from build123d import *

# Parameters (mm, degrees)
BOSS_EXTRUDE1_DEPTH      = 3
SKETCH2_W                = 3
SKETCH2_H                = 34
BOSS_EXTRUDE2_DEPTH      = 17
BOSS_EXTRUDE2_DEPTH_BACK = 3
SKETCH3_W                = 22.5
SKETCH3_H                = 29.060921084
CUT_EXTRUDE1_DEPTH       = 18
CUT_EXTRUDE2_DEPTH       = 1.5
CHAMFER1_SIZE            = 10
CHAMFER2_SIZE            = 1.5
CHAMFER2_SIZE2           = 2.223841453
SKETCH7_W                = 31
SKETCH7_H                = 2
BOSS_EXTRUDE3_DEPTH      = 2
BOSS_EXTRUDE3_DEPTH_BACK = 3
SKETCH9_W                = 0.5
SKETCH9_H                = 11.560921084
CUT_EXTRUDE4_DEPTH       = 10
CHAMFER3_SIZE            = 1.5
CUT_EXTRUDE6_START       = -16.5
SKETCH11_W               = 3
SKETCH11_H               = 5
CUT_EXTRUDE6_DEPTH       = 16.5
CHAMFER9_SIZE            = 2
CHAMFER10_SIZE           = 3.5
FILLET2_R                = 2


with BuildPart() as part:
    # Sketch1 → Boss-Extrude1 (new body)
    with BuildSketch(Plane.XY):
        with BuildLine():
            Line((38, 38.915798387), (-38, 38.915798387))
            Line((-38, 38.915798387), (-38, 9.854877303))
            Line((-38, 9.854877303), (-34.5, 9.854877303))
            Line((-34.5, 9.854877303), (-34.5, 15.915798387))
            Line((-34.5, 15.915798387), (-34.5, 21.415798387))
            Line((-34.5, 21.415798387), (-29, 21.415798387))
            Line((-29, 21.415798387), (-21, 21.415798387))
            ThreePointArc((-21, 21.415798387), (-17.110912703, 19.804885683), (-15.5, 15.915798387))
            Line((-15.5, 15.915798387), (-15.5, 9.854877303))
            Line((-15.5, 9.854877303), (15.5, 9.854877303))
            Line((15.5, 9.854877303), (15.5, 15.915798387))
            ThreePointArc((15.5, 15.915798387), (17.110912703, 19.804885683), (21, 21.415798387))
            Line((21, 21.415798387), (29, 21.415798387))
            ThreePointArc((29, 21.415798387), (32.889087297, 19.804885683), (34.5, 15.915798387))
            Line((34.5, 15.915798387), (34.5, 9.854877303))
            Line((34.5, 9.854877303), (38, 9.854877303))
            Line((38, 9.854877303), (38, 38.915798387))
        make_face()
        with BuildLine():
            Line((-10.5, 33.665798387), (-5.5, 33.665798387))
            ThreePointArc((-5.5, 33.665798387), (-3.75, 31.915798387), (-5.5, 30.165798387))
            Line((-5.5, 30.165798387), (-10.5, 30.165798387))
            ThreePointArc((-10.5, 30.165798387), (-12.25, 31.915798387), (-10.5, 33.665798387))
        make_face(mode=Mode.SUBTRACT)
        with BuildLine():
            Line((5.5, 33.665798387), (10.5, 33.665798387))
            ThreePointArc((10.5, 33.665798387), (12.25, 31.915798387), (10.5, 30.165798387))
            Line((10.5, 30.165798387), (5.5, 30.165798387))
            ThreePointArc((5.5, 30.165798387), (3.75, 31.915798387), (5.5, 33.665798387))
        make_face(mode=Mode.SUBTRACT)
        with BuildLine():
            Line((5.5, 17.665798387), (10.5, 17.665798387))
            ThreePointArc((10.5, 17.665798387), (12.25, 15.915798387), (10.5, 14.165798387))
            Line((10.5, 14.165798387), (5.5, 14.165798387))
            ThreePointArc((5.5, 14.165798387), (3.75, 15.915798387), (5.5, 17.665798387))
        make_face(mode=Mode.SUBTRACT)
        with BuildLine():
            Line((-10.5, 17.665798387), (-5.5, 17.665798387))
            ThreePointArc((-5.5, 17.665798387), (-3.75, 15.915798387), (-5.5, 14.165798387))
            Line((-5.5, 14.165798387), (-10.5, 14.165798387))
            ThreePointArc((-10.5, 14.165798387), (-12.25, 15.915798387), (-10.5, 17.665798387))
        make_face(mode=Mode.SUBTRACT)
    extrude(amount=BOSS_EXTRUDE1_DEPTH)

    # Sketch2 → Boss-Extrude2 (add, two sides)
    with BuildSketch(Plane.XY.offset(3)) as boss_extrude2_sk:
        with Locations((-36.5, 21.915798387)):
            Rectangle(SKETCH2_W, SKETCH2_H)
    extrude(amount=BOSS_EXTRUDE2_DEPTH)
    extrude(boss_extrude2_sk.sketch, amount=-BOSS_EXTRUDE2_DEPTH_BACK)

    # Sketch3 → Cut-Extrude1 (cut)
    with BuildSketch(Plane.XY.offset(3)):
        with Locations((26.75, 24.385337845)):
            Rectangle(SKETCH3_W, SKETCH3_H)
    extrude(amount=-CUT_EXTRUDE1_DEPTH, mode=Mode.SUBTRACT)

    # Sketch4 → Cut-Extrude2 (cut)
    with BuildSketch(Plane(origin=(0, 0, 0), x_dir=(-1, 0, 0), z_dir=(0, 0, -1))):
        with BuildLine():
            Line((4.8, 35.115798387), (11.2, 35.115798387))
            ThreePointArc((11.2, 35.115798387), (14.4, 31.915798387), (11.2, 28.715798387))
            Line((11.2, 28.715798387), (4.8, 28.715798387))
            ThreePointArc((4.8, 28.715798387), (1.6, 31.915798387), (4.8, 35.115798387))
        make_face()
        with BuildLine():
            Line((-11.2, 35.115798387), (-4.8, 35.115798387))
            ThreePointArc((-4.8, 35.115798387), (-1.6, 31.915798387), (-4.8, 28.715798387))
            Line((-4.8, 28.715798387), (-11.2, 28.715798387))
            ThreePointArc((-11.2, 28.715798387), (-14.4, 31.915798387), (-11.2, 35.115798387))
        make_face()
        with BuildLine():
            Line((4.8, 19.115798387), (11.2, 19.115798387))
            ThreePointArc((11.2, 19.115798387), (14.4, 15.915798387), (11.2, 12.715798387))
            Line((11.2, 12.715798387), (4.8, 12.715798387))
            ThreePointArc((4.8, 12.715798387), (1.6, 15.915798387), (4.8, 19.115798387))
        make_face()
        with BuildLine():
            Line((-11.2, 19.115798387), (-4.8, 19.115798387))
            ThreePointArc((-4.8, 19.115798387), (-1.6, 15.915798387), (-4.8, 12.715798387))
            Line((-4.8, 12.715798387), (-11.2, 12.715798387))
            ThreePointArc((-11.2, 12.715798387), (-14.4, 15.915798387), (-11.2, 19.115798387))
        make_face()
    extrude(amount=-CUT_EXTRUDE2_DEPTH, mode=Mode.SUBTRACT)

    # Chamfer1
    chamfer1_edges = [part.edges().sort_by_distance(p)[0] for p in [
        (-36.5, 38.915798387, 20),
    ]]
    chamfer(chamfer1_edges, length=CHAMFER1_SIZE)

    # Chamfer2
    chamfer2_edges = [part.edges().sort_by_distance(p)[0] for p in [
        (0, 9.854877303, 0),
    ]]
    chamfer2_side = [part.faces().sort_by_distance(p)[0] for p in [
        (-11.889403283, 26.058636035, 0),
    ]]
    chamfer(chamfer2_edges, length=CHAMFER2_SIZE, length2=CHAMFER2_SIZE2, reference=chamfer2_side[0])

    # Sketch7 → Boss-Extrude3 (add, two sides)
    with BuildSketch(Plane.XY.offset(3)) as boss_extrude3_sk:
        with Locations((0, 39.415798387)):
            Rectangle(SKETCH7_W, SKETCH7_H)
    extrude(amount=BOSS_EXTRUDE3_DEPTH)
    extrude(boss_extrude3_sk.sketch, amount=-BOSS_EXTRUDE3_DEPTH_BACK)

    # Sketch9 → Cut-Extrude4 (cut)
    with BuildSketch(Plane(origin=(0, 0, 0), x_dir=(-1, 0, 0), z_dir=(0, 0, -1))):
        with Locations((34.75, 15.635337845)):
            Rectangle(SKETCH9_W, SKETCH9_H)
    extrude(amount=-CUT_EXTRUDE4_DEPTH, mode=Mode.SUBTRACT)

    # Chamfer3
    chamfer3_edges = [part.edges().sort_by_distance(p)[0] for p in [
        (0, 40.415798387, 0),
    ]]
    chamfer(chamfer3_edges, length=CHAMFER3_SIZE)

    # Sketch11 → Cut-Extrude6 (cut)
    with BuildSketch(Plane(origin=(0, 4.915798387, 0), x_dir=(-1, 0, 0), z_dir=(0, -1, 0)).offset(CUT_EXTRUDE6_START)):
        with Locations((36.5, -2.5)):
            Rectangle(SKETCH11_W, SKETCH11_H)
    extrude(amount=CUT_EXTRUDE6_DEPTH, mode=Mode.SUBTRACT)

    # Chamfer9
    chamfer9_edges = [part.edges().sort_by_distance(p)[0] for p in [
        (-35, 30.165798387, 3),
    ]]
    chamfer(chamfer9_edges, length=CHAMFER9_SIZE)

    # Chamfer10
    chamfer10_edges = [part.edges().sort_by_distance(p)[0] for p in [
        (-38, 30.165798387, 0),
    ]]
    chamfer(chamfer10_edges, length=CHAMFER10_SIZE)

    # Fillet2
    fillet2_edges = [part.edges().sort_by_distance(p)[0] for p in [
        (-36.5, 21.415798387, 5),
        (-36.5, 38.915798387, 10),
        (-36.5, 28.915798387, 20),
        (-36.5, 4.915798387, 20),
        (-36.5, 4.915798387, 5),
        (-15.5, 39.415798387, 5),
        (15.5, 39.415798387, 5),
    ]]
    fillet(fillet2_edges, radius=FILLET2_R)


solid = part.part
Verification items for the finished model (mm, model axes). A direction names the side the tool comes from. Coordinates: 2 decimals unless noted, no trailing zeros. Order: outer loops, then holes, each group sorted by start corner. A loop starts at its lowest first (then second) coordinate and runs counter-clockwise, first axis right, second up. Notation, with made-up numbers: (6.25, -14.75) -> (29.25, -14.75) arc R21 ccw to (29.25, 4.25) -> close; hole circle Ø10 at (-30, 58). An arc over 180 degrees is marked (long way). Put each result on its own line as item: value. Start each with the question number.
1. Cross-section at B-B, the plane y = 31.5. Record the boundary of the cut face in (x, z).
2. Cross-section at D-D, the plane x = -30. Record the boundary of the cut face in (y, z), then the cut area to 3 significant figures.
3. Cross-section at A-A, the plane x = 0.5. Record the boundary of the cut face in (y, z), then the cut area to 3 significant figures.
4. Access from +Z, -Z, +X, -X, +Y, -Y to the whole of each face (thin tool, end or side, straight path). Record for faces 3 (the flat face through (0, 38.416, 4)), 4 (the cylindrical face through (14.4, 15.85, 0.74)), 5 (the flat face through (-15.5, 40, 2)), 6 (the flat face through (-8, 14.166, 2)).
5. Mould release check, pull along Z, two halves, no side actions. Record for faces 1 (the cylindrical face through (12.25, 15.95, 2.24)), 2 (the cylindrical face through (-36.48, 5.52, 19.43)): released by +Z, released by -Z, zero draft, split by the parting line, or undercut.
6. Go/stop test with flat-tipped pins: pin 1 Ø8.5 at (x, y) = (-17.5, 22.5) entering from +Z; pin 2 Ø6 at (y, z) = (12.5, 16.5) entering from +X; pin 3 Ø1.2 at (x, z) = (-9, 2) entering from -Y. Record where each tip stops, or that it passes through.
7. Material ranges on L1, parallel to Y at x = -9, z = 2.5; L2, parallel to Z at x = -10.5, y = 26.5; L3, parallel to X at y = 17, z = 16.5, recorded low to high. Write a range as [from, to].
8. Cross-section at C-C, the plane z = 13.25. Record the boundary of the cut face in (x, y), then the cut area to 4 significant figures.
Computed:
1. outline: (-38, 3.5) -> (-34.5, 0) -> (-14.37, 0) -> (-14.37, 1.5) -> (-12.2, 1.5) -> (-12.2, 3) -> (-33, 3) -> (-35, 5) -> (-35, 17.42) -> (-38, 17.42) -> close; (-3.8, 1.5) -> (-1.63, 1.5) -> (-1.63, 0) -> (1.63, 0) -> (1.63, 1.5) -> (3.8, 1.5) -> (3.8, 3) -> (-3.8, 3) -> close; (12.2, 1.5) -> (14.37, 1.5) -> (14.37, 0) -> (15.5, 0) -> (15.5, 3) -> (12.2, 3) -> close
2. outline: (21.42, 0) -> (38.92, 0) -> (38.92, 3) -> (21.42, 3) -> close
2. area: 52.5 mm2
3. outline: (9.85, 2.22) -> (11.35, 0) -> (38.92, 0) -> (40.42, 1.5) -> (40.42, 5) -> (38.42, 5) -> (38.42, 3) -> (9.85, 3) -> close
3. area: 92.9 mm2
4. face 3: +Z, +X, -Y
4. face 4: -Z
4. face 5: +Z, -Z, -X, +Y
4. face 6: +Z, -Z
5. face 1: zero draft
5. face 2: released by +Z
6. pin 1: z = 3
6. pin 2: x = -35
6. pin 3: y = 9.85
7. L1: [9.85, 14.17], [17.67, 30.17], [33.67, 40.42]
7. L2: [0, 3]
7. L3: [-38, -35]
8. outline: (-38, 4.92) -> (-35, 4.92) -> (-35, 35.67) -> (-38, 35.67) -> close
8. area: 92.25 mm2
